CAD build for the part. Positions are in the model's coordinates, mm. A direction names the side the tool comes from. Give positions to 0.01 mm unless a question says otherwise; leave off trailing zeros. Write each loop counter-clockwise with the first axis right and the second up, starting at its lowest first coordinate (ties: lowest second). Pieces come first, ordered by that corner, then holes. Notation, with made-up numbers: (33.25, 36) - (40.25, 36) arc R13 ccw to (40.25, 59) - close; hole circle Ø4 at (12.5, 20). An arc over 180 degrees is marked (long way). Answer as a JSON object with one key per item and string values.
from build123d import *

# Parameters (mm, degrees)
MODEL_R             = 2.5
MODEL_R_2           = 3
BOSS_EXTRUDE1_DEPTH = 60


with BuildPart() as part:
    # Model → Boss-Extrude1 (new body)
    with BuildSketch(Plane.XY):
        with BuildLine():
            Line((-27.5, 3.25), (-30, 3.25))
            Line((-30, 3.25), (-30, 14))
            ThreePointArc((-30, 14), (-29.707106781, 14.707106781), (-29, 15))
            Line((-29, 15), (-18.25, 15))
            Line((-18.25, 15), (-18.25, 12.5))
            Line((-18.25, 12.5), (-20.25, 12.5))
            Line((-20.25, 12.5), (-20.25, 6.643928679))
            ThreePointArc((-20.25, 6.643928679), (-15, 4.5), (-9.75, 6.643928679))
            Line((-9.75, 6.643928679), (-9.75, 12.5))
            Line((-9.75, 12.5), (-11.75, 12.5))
            Line((-11.75, 12.5), (-11.75, 15))
            Line((-11.75, 15), (11.75, 15))
            Line((11.75, 15), (11.75, 12.5))
            Line((11.75, 12.5), (9.75, 12.5))
            Line((9.75, 12.5), (9.75, 6.643928679))
            ThreePointArc((9.75, 6.643928679), (15, 4.5), (20.25, 6.643928679))
            Line((20.25, 6.643928679), (20.25, 12.5))
            Line((20.25, 12.5), (18.25, 12.5))
            Line((18.25, 12.5), (18.25, 15))
            Line((18.25, 15), (29, 15))
            ThreePointArc((29, 15), (29.707106781, 14.707106781), (30, 14))
            Line((30, 14), (30, 3.25))
            Line((30, 3.25), (27.5, 3.25))
            Line((27.5, 3.25), (27.5, 5.25))
            Line((27.5, 5.25), (21.643928679, 5.25))
            ThreePointArc((21.643928679, 5.25), (19.5, 0), (21.643928679, -5.25))
            Line((21.643928679, -5.25), (27.5, -5.25))
            Line((27.5, -5.25), (27.5, -3.25))
            Line((27.5, -3.25), (30, -3.25))
            Line((30, -3.25), (30, -14))
            ThreePointArc((30, -14), (29.707106781, -14.707106781), (29, -15))
            Line((29, -15), (18.25, -15))
            Line((18.25, -15), (18.25, -12.5))
            Line((18.25, -12.5), (20.25, -12.5))
            Line((20.25, -12.5), (20.25, -6.643928679))
            ThreePointArc((20.25, -6.643928679), (15, -4.5), (9.75, -6.643928679))
            Line((9.75, -6.643928679), (9.75, -12.5))
            Line((9.75, -12.5), (11.75, -12.5))
            Line((11.75, -12.5), (11.75, -15))
            Line((11.75, -15), (-11.75, -15))
            Line((-11.75, -15), (-11.75, -12.5))
            Line((-11.75, -12.5), (-9.75, -12.5))
            Line((-9.75, -12.5), (-9.75, -6.643928679))
            ThreePointArc((-9.75, -6.643928679), (-15, -4.5), (-20.25, -6.643928679))
            Line((-20.25, -6.643928679), (-20.25, -12.5))
            Line((-20.25, -12.5), (-18.25, -12.5))
            Line((-18.25, -12.5), (-18.25, -15))
            Line((-18.25, -15), (-29, -15))
            ThreePointArc((-29, -15), (-29.707106781, -14.707106781), (-30, -14))
            Line((-30, -14), (-30, -3.25))
            Line((-30, -3.25), (-27.5, -3.25))
            Line((-27.5, -3.25), (-27.5, -5.25))
            Line((-27.5, -5.25), (-21.643928679, -5.25))
            ThreePointArc((-21.643928679, -5.25), (-19.5, 0), (-21.643928679, 5.25))
            Line((-21.643928679, 5.25), (-27.5, 5.25))
            Line((-27.5, 5.25), (-27.5, 3.25))
        make_face()
        with Locations((-15, 0)):
            Circle(MODEL_R, mode=Mode.SUBTRACT)
        with Locations((-25, 10.531430074)):
            Circle(MODEL_R_2, mode=Mode.SUBTRACT)
        with Locations((-25.399251578, -9.468569926)):
            Circle(MODEL_R_2, mode=Mode.SUBTRACT)
        with Locations((25.399251578, -9.468569926)):
            Circle(MODEL_R_2, mode=Mode.SUBTRACT)
        with Locations((15, 0)):
            Circle(MODEL_R, mode=Mode.SUBTRACT)
        with Locations((25, 10.531430074)):
            Circle(MODEL_R_2, mode=Mode.SUBTRACT)
        with BuildLine():
            Line((6.5, 12), (-6.5, 12))
            ThreePointArc((-6.5, 12), (-7.914213562, 11.414213562), (-8.5, 10))
            Line((-8.5, 10), (-8.5, -10))
            ThreePointArc((-8.5, -10), (-7.914213562, -11.414213562), (-6.5, -12))
            Line((-6.5, -12), (6.5, -12))
            ThreePointArc((6.5, -12), (7.914213562, -11.414213562), (8.5, -10))
            Line((8.5, -10), (8.5, 10))
            ThreePointArc((8.5, 10), (7.914213562, 11.414213562), (6.5, 12))
        make_face(mode=Mode.SUBTRACT)
    extrude(amount=BOSS_EXTRUDE1_DEPTH)


solid = part.part
(1) Pull direction Y, two halves, no side cores. Call faces 6 (the face through (24, -15, 30)), 7 (the face through (30, -9, 30)), 8 (the face through (-27.5, -4, 30)): pulls with the +Y half, pulls with the -Y half, needs draft (parallel to the pull), parting line crosses it, or undercut.
Answer key:
{"face 6": "pulls with the -Y half", "face 7": "needs draft", "face 8": "undercut"}
(2) Flat gauge pins, fed straight in: P1, Ø16, axis at y = -2, z = 26, coming from the -X side; P2, Ø4, axis at x = 15, z = 43.5, coming from the +Y side. Where does each tip first touch, or does it go through?
Answer key:
{"P1": "stops at x = -30", "P2": "stops at y = 4.77"}
(3) Saw through at C-C, the plane y = -11. Give the cut face in (x, z).
Answer key:
{"outline": "(-30, 0) - (-27.98, 0) - (-27.98, 60) - (-30, 60) - close; (-22.82, 0) - (-20.25, 0) - (-20.25, 60) - (-22.82, 60) - close; (-9.75, 0) - (-8.23, 0) - (-8.23, 60) - (-9.75, 60) - close; (8.23, 0) - (9.75, 0) - (9.75, 60) - (8.23, 60) - close; (20.25, 0) - (22.82, 0) - (22.82, 60) - (20.25, 60) - close; (27.98, 0) - (30, 0) - (30, 60) - (27.98, 60) - close"}
(4) Saw through at D-D, the plane x = 25. Give the cut face in (y, z).
Answer key:
{"outline": "(-15, 0) - (-12.44, 0) - (-12.44, 60) - (-15, 60) - close; (-6.5, 0) - (-5.25, 0) - (-5.25, 60) - (-6.5, 60) - close; (5.25, 0) - (7.53, 0) - (7.53, 60) - (5.25, 60) - close; (13.53, 0) - (15, 0) - (15, 60) - (13.53, 60) - close"}
(5) Saw through at B-B, the plane y = 0. Give the cut face in (x, z).
Answer key:
{"outline": "(-19.5, 0) - (-17.5, 0) - (-17.5, 60) - (-19.5, 60) - close; (-12.5, 0) - (-8.5, 0) - (-8.5, 60) - (-12.5, 60) - close; (8.5, 0) - (12.5, 0) - (12.5, 60) - (8.5, 60) - close; (17.5, 0) - (19.5, 0) - (19.5, 60) - (17.5, 60) - close"}
(6) Saw through at A-A, the plane x = -15. Give the cut face in (y, z).
Answer key:
{"outline": "(-4.5, 0) - (-2.5, 0) - (-2.5, 60) - (-4.5, 60) - close; (2.5, 0) - (4.5, 0) - (4.5, 60) - (2.5, 60) - close"}
(7) 3-axis set-ups, long thin cutter, end or side, ignore diameter. For faces 1 (the face through (29, 3.25, 30)), 2 (the face through (-29, -3.25, 30)), 3 (the face through (-20.25, 10, 30)), 4 (the face through (-11.75, -14, 30)), 5 (the face through (-11.75, 14, 30)): which of +Z, -Z, +X, -X, +Y, -Y reach the whole face in a straight line?
Answer key:
{"face 1": "+Z, -Z, +X", "face 2": "+Z, -Z, -X", "face 3": "+Z, -Z", "face 4": "+Z, -Z, -Y", "face 5": "+Z, -Z, +Y"}
(8) Probe L1, parallel to X at y = 6.75, z = 23; L2, parallel to X at y = 10.25, z = 14; L3, parallel to X at y = 1.25, z = 44.5. List the from-to ranges inside material, lowest first. Write a range as [from, to].
Answer key:
{"L1": "x = [-30, -20.25], [-9.75, -8.5], [8.5, 9.75], [20.25, 30]", "L2": "x = [-30, -27.99], [-22.01, -20.25], [-9.75, -8.48], [8.48, 9.75], [20.25, 22.01], [27.99, 30]", "L3": "x = [-19.6, -17.17], [-12.83, -8.5], [8.5, 12.83], [17.17, 19.6]"}
